Here's how the part is built. I have some questions about the finished solid (model axes, mm). Face numbers are marked on the shaded views. A direction names the side the tool comes from. Give positions to 0.01 mm unless a question says otherwise; leave off trailing zeros. Use CSV: the item, a comma, the result in double quotes. Start each with the question number.
(1) For pin 1 Ø8 at (y, z) = (-6, -19) entering from -X; pin 2 Ø1 at (x, z) = (-30.5, -14.5) entering from -Y; pin 3 Ø4 at (x, y) = (43, 11) entering from +Z, each with a flat end and sliding along its axis, tell me the tip position at first contact or that it passes through.
(2) I need wall thicknesses on L1, parallel to X at y = 14.5, z = -4.5; L2, parallel to Y at x = -35, z = 2; L3, parallel to Z at x = 39.5, y = 3. Which ranges of each line are inside material? Lowest first, please. Write a range as [from, to].
(3) If we mould it in two halves opening along X, with no side actions, what happens to the marked faces 1, 2 and 3? For each: pulls with the +X half, pulls with the -X half, needs draft (parallel to the pull), parting line crosses it, or undercut.
(4) Which directions (+Z, -Z, +X, -X, +Y, -Y) give clear straight access to the entire face, cutting with the end or side of a thin tool? Please do the marked faces 4, 5 and 6.
(5) Suppose I cut it at A-A on z = 2.54. Give the number of separate pieces and of enclosed holes in the cut face, plus the area to 3 significant figures.
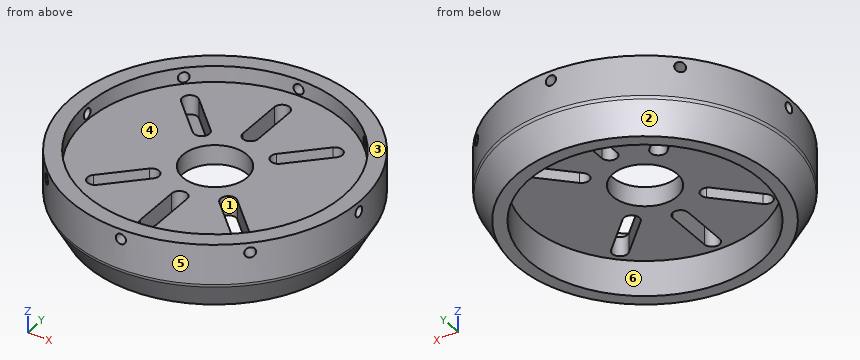
from build123d import *

# Parameters (mm, degrees)
CUT_EXTRUDE1_DEPTH = 84.656279501
CIRPATTERN1_COUNT  = 8
SKETCH3_R          = 2.032
CUT_EXTRUDE2_DEPTH = 84.656279501
CIRPATTERN2_COUNT  = 8
FILLET1_R          = 2.54


with BuildPart() as part:
    # Sketch1 → Revolve1 (revolve)
    with BuildSketch(Plane(origin=(0, 0, 0), x_dir=(0, 0, -1), z_dir=(1, 0, 0)), mode=Mode.PRIVATE) as revolve1_sk:
        Polygon((0, 12.7), (0, 50.8), (-6.35, 50.8), (-6.35, 57.15), (10.16, 57.15), (21.59, 50.8), (21.59, 45.72), (7.62, 45.72), (7.62, 12.7), align=None)
    revolve(revolve1_sk.sketch.rotate(Axis((0, 0, 0), (0, 0, -1)), 90), axis=Axis((0, 0, 0), (0, 0, -1)))

    # Sketch2 → Cut-Extrude1 (cut, through all)
    with BuildSketch(Plane.XY):
        with BuildLine():
            Line((-3.048, 21.59), (-3.048, 40.64))
            ThreePointArc((-3.048, 40.64), (0, 43.688), (3.048, 40.64))
            Line((3.048, 40.64), (3.048, 21.59))
            ThreePointArc((3.048, 21.59), (0, 18.542), (-3.048, 21.59))
        make_face()
    cut_extrude1 = extrude(amount=-CUT_EXTRUDE1_DEPTH, mode=Mode.SUBTRACT)

    # CirPattern1: Cut-Extrude1 ×8 about axis, 2 skipped
    cirpattern1_axis = Axis((0, 0, 0), (0, 0, -1))
    add([cut_extrude1.rotate(cirpattern1_axis, i * 360 / CIRPATTERN1_COUNT) for i in range(1, CIRPATTERN1_COUNT) if i not in (2, 6)], mode=Mode.SUBTRACT)

    # Sketch3 → Cut-Extrude2 (cut, through all)
    with BuildSketch(Plane(origin=(0, 0, 0), x_dir=(1, 0, 0), z_dir=(0, 1, 0))):
        with Locations(Location((0, -2.54, 0), (0, 0, 270))):
            Circle(SKETCH3_R)
    cut_extrude2 = extrude(amount=-CUT_EXTRUDE2_DEPTH, mode=Mode.SUBTRACT)

    # CirPattern2: Cut-Extrude2 ×8 about axis
    cirpattern2_axis = Axis((0, 0, 0), (0, 0, 1))
    for i in range(1, CIRPATTERN2_COUNT):
        add(cut_extrude2.rotate(cirpattern2_axis, i * 360 / CIRPATTERN2_COUNT), mode=Mode.SUBTRACT)

    # Fillet1
    fillet1_edges = [part.edges().sort_by_distance(p)[0] for p in [
        (-57.15, 0, -10.16),
    ]]
    fillet(fillet1_edges, radius=FILLET1_R)


solid = part.part
Geometry says:
1,pin 1,"x = -54.17"
1,pin 2,"y = -45.92"
1,pin 3,"z = 0"
2,L1,"[-55.28, -18.81], [-12.32, 12.32], [18.81, 55.28]"
2,L2,"[-45.18, -37.77], [37.77, 45.18]"
2,L3,"[-7.62, 0]"
3,face 1,"undercut"
3,face 2,"parting line crosses it"
3,face 3,"needs draft"
4,face 4,"+Z"
4,face 5,"+Z, -Z"
4,face 6,"-Z"
5,separate pieces,"8"
5,enclosed holes,"0"
5,area,"1,950 mm²"
